```python
from build123d import *

# Parameters (mm, degrees)
SKETCH1_W           = 25.4
SKETCH1_H           = 92.71
BOSS_EXTRUDE1_DEPTH = 5.08
SKETCH3_W           = 13.208
SKETCH3_H           = 5.08
BOSS_EXTRUDE3_DEPTH = 11.938
SKETCH5_R           = 1.905
CUT_EXTRUDE2_DEPTH  = 6.08
SKETCH7_W           = 25.4
SKETCH7_H           = 92.71
BOSS_EXTRUDE4_DEPTH = 1.778
SKETCH8_R           = 3.937
CUT_EXTRUDE3_DEPTH  = 1.27
SKETCH10_R          = 3.81
BOSS_EXTRUDE5_DEPTH = 3.81
SKETCH11_W          = 13.208
SKETCH11_H          = 5.08
BOSS_EXTRUDE6_DEPTH = 7.62
CUT_EXTRUDE4_DEPTH  = 6.08
FILLET1_R           = 0.635
CUT_EXTRUDE7_DEPTH  = 7.62
CUT_EXTRUDE8_DEPTH  = 7.8580001
SKETCH17_W          = 12.7
SKETCH17_H          = 82.55
BOSS_EXTRUDE7_DEPTH = 1.524


with BuildPart() as part:
    # Sketch1 → Boss-Extrude1 (new body)
    with BuildSketch(Plane.XY):
        with Locations((-20.361983471, -4.405640496)):
            Rectangle(SKETCH1_W, SKETCH1_H)
    extrude(amount=BOSS_EXTRUDE1_DEPTH)

    # Sketch3 → Boss-Extrude3 (add)
    with BuildSketch(Plane.XZ.offset(50.760640496)):
        with Locations((-20.361983471, 2.54)):
            Rectangle(SKETCH3_W, SKETCH3_H)
    extrude(amount=BOSS_EXTRUDE3_DEPTH)

    # Sketch5 → Cut-Extrude2 (cut, through all)
    with BuildSketch(Plane.XY.offset(5.08)):
        with Locations((-20.361983471, -56.094640496)):
            Circle(SKETCH5_R)
        with BuildLine():
            Line((-23.722087636, -58.380640496), (-26.965983471, -58.380640496))
            Line((-26.965983471, -58.380640496), (-26.965983471, -62.698640496))
            Line((-26.965983471, -62.698640496), (-13.757983471, -62.698640496))
            Line((-13.757983471, -62.698640496), (-13.757983471, -58.380640496))
            Line((-13.757983471, -58.380640496), (-17.001879306, -58.380640496))
            ThreePointArc((-17.001879306, -58.380640496), (-20.361983471, -60.158640496), (-23.722087636, -58.380640496))
        make_face()
    extrude(amount=-CUT_EXTRUDE2_DEPTH, mode=Mode.SUBTRACT)

    # Sketch7 → Boss-Extrude4 (add)
    with BuildSketch(Plane.XY.offset(5.08)):
        with Locations((-20.361983471, -4.405640496)):
            Rectangle(SKETCH7_W, SKETCH7_H)
    extrude(amount=BOSS_EXTRUDE4_DEPTH)

    # Sketch8 → Cut-Extrude3 (cut)
    with BuildSketch(Plane.XY.offset(6.858)):
        with Locations((-20.361983471, -42.378640496)):
            Circle(SKETCH8_R)
        with Locations((-20.361983471, -4.278640496)):
            Circle(SKETCH8_R)
        with Locations((-20.361983471, 33.821359504)):
            Circle(SKETCH8_R)
    extrude(amount=-CUT_EXTRUDE3_DEPTH, mode=Mode.SUBTRACT)

    # Sketch10 → Boss-Extrude5 (add)
    with BuildSketch(Plane.XY.offset(5.588)):
        with Locations((-20.361983471, -42.378640496)):
            Circle(SKETCH10_R)
        with Locations((-20.361983471, -4.278640496)):
            Circle(SKETCH10_R)
        with Locations((-20.361983471, 33.821359504)):
            Circle(SKETCH10_R)
    extrude(amount=BOSS_EXTRUDE5_DEPTH)

    # Sketch11 → Boss-Extrude6 (add)
    with BuildSketch(Plane(origin=(0, 41.949359504, 0), x_dir=(1, 0, 0), z_dir=(0, 1, 0))):
        with Locations((-20.361983471, -2.54)):
            Rectangle(SKETCH11_W, SKETCH11_H)
    extrude(amount=BOSS_EXTRUDE6_DEPTH)

    # Sketch12 → Cut-Extrude4 (cut, through all)
    with BuildSketch(Plane.XY.offset(5.08)):
        Polygon((-23.155983471, 49.569359504), (-20.361983471, 46.013359504), (-17.567983471, 49.569359504), align=None)
    extrude(amount=-CUT_EXTRUDE4_DEPTH, mode=Mode.SUBTRACT)

    # Fillet1
    fillet1_edges = [part.edges().sort_by_distance(p)[0] for p in [
        (-20.361983471, 46.013359504, 2.54),
        (-26.965983471, 49.569359504, 2.54),
        (-13.757983471, 49.569359504, 2.54),
    ]]
    fillet(fillet1_edges, radius=FILLET1_R)

    # Sketch14 → Cut-Extrude7 (cut)
    with BuildSketch(Plane.XY.offset(6.858)):
        with BuildLine():
            Line((-13.757983471, 41.949359504), (-7.661983471, 41.949359504))
            Line((-7.661983471, 41.949359504), (-7.661983471, -4.405640496))
            add(Edge.make_bspline(
                [(-13.757983471, 41.949359504), (-7.661983471, 18.771859504), (-7.661983471, -4.405640496)],
                knots=[0, 0, 0, 0.5, 0.5, 0.5], degree=2))
        make_face()
        with BuildLine():
            Line((-33.061983471, -4.405640496), (-33.061983471, 41.949359504))
            Line((-33.061983471, 41.949359504), (-26.965983471, 41.949359504))
            add(Edge.make_bspline(
                [(-26.965983471, 41.949359504), (-33.061983471, 18.771859504), (-33.061983471, -4.405640496)],
                knots=[0, 0, 0, 0.5, 0.5, 0.5], degree=2))
        make_face()
    extrude(amount=-CUT_EXTRUDE7_DEPTH, mode=Mode.SUBTRACT)

    # Sketch16 → Cut-Extrude8 (cut, through all)
    with BuildSketch(Plane.XY.offset(6.858)):
        with BuildLine():
            Line((-33.061983471, -4.405640496), (-33.061983471, -50.760640496))
            Line((-33.061983471, -50.760640496), (-26.965983471, -50.760640496))
            add(Edge.make_bspline(
                [(-33.061983471, -4.405640496), (-33.061983471, -27.583140496), (-26.965983471, -50.760640496)],
                knots=[0.5, 0.5, 0.5, 1, 1, 1], degree=2))
        make_face()
        with BuildLine():
            Line((-7.661983471, -4.405640496), (-7.661983471, -50.760640496))
            Line((-7.661983471, -50.760640496), (-13.757983471, -50.760640496))
            add(Edge.make_bspline(
                [(-13.757983471, -50.760640496), (-7.661983471, -27.583140496), (-7.661983471, -4.405640496)],
                knots=[0, 0, 0, 0.5, 0.5, 0.5], degree=2))
        make_face()
    extrude(amount=-CUT_EXTRUDE8_DEPTH, mode=Mode.SUBTRACT)

    # Sketch17 → Boss-Extrude7 (add)
    with BuildSketch(Plane(origin=(0, 0, 0), x_dir=(-1, 0, 0), z_dir=(0, 0, -1))):
        with Locations((20.361983471, -4.405640496)):
            Rectangle(SKETCH17_W, SKETCH17_H)
    extrude(amount=BOSS_EXTRUDE7_DEPTH)


solid = part.part
```
Source: CAD feature listing. Evaluate the final solid. Frame: model axes, mm. A direction names the side the tool comes from. Round coordinates to 2 decimals unless told otherwise and drop trailing zeros. Use CSV: the item, a comma, the result in double quotes. Start each with the question number.
Q1. Pull-direction query (X, two-part tool) for faces 5 (the face through (-18.73, 48.09, 2.58)), 6 (the face through (-26.966, -55, 3)), 7 (the face through (-20, 34, 9.398)); classes: +X half, -X half, draft (parallel to the pull), parting line (faces both ways), or undercut.
Q2. First-contact query: P1, Ø0.8, axis at y = 15, z = -1, coming from the -X side; P2, Ø3, axis at x = -18.5, y = -56.5, coming from the +Z side; P3, Ø0.8, axis at x = -21.5, z = -1, coming from the -Y side. Flat tips, straight axial feed; report the tip coordinate or a pass-through.
Q3. Access query for faces 1 (the face through (-20.86, -38.6, 7.47)), 2 (the face through (-13.758, -55, 3)), 3 (the face through (-26.966, 45, 3)), 4 (the face through (-20, 41.949, 6)). Directions: +Z, -Z, +X, -X, +Y, -Y. A direction counts if a zero-diameter tool reaches every point of the face in a straight line with its end or side. Return the directions, or none.
Q4. Line query: line 1 (Y direction, x = -20, z = 8.75); line 2 (Y direction, x = -20.25, z = 1); line 3 (Z direction, x = -17.5, y = 45). Output: solid intervals per line, ascending. Write a range as from..to.
Results found:
1,face 5,"undercut"
1,face 6,"-X half"
1,face 7,"draft"
2,P1,"x = -26.71"
2,P2,"z = 5.08"
2,P3,"y = -45.68"
3,face 1,"+Z"
3,face 2,"+Z, -Z, +X, -Y"
3,face 3,"+Z, -Z, -X, +Y"
3,face 4,"+Z, +X, -X, +Y"
4,line 1,"-46.17..-38.59, -8.07..-0.49, 30.03..37.61"
4,line 2,"-60.16..-58, -54.19..46.42"
4,line 3,"0..5.08"
